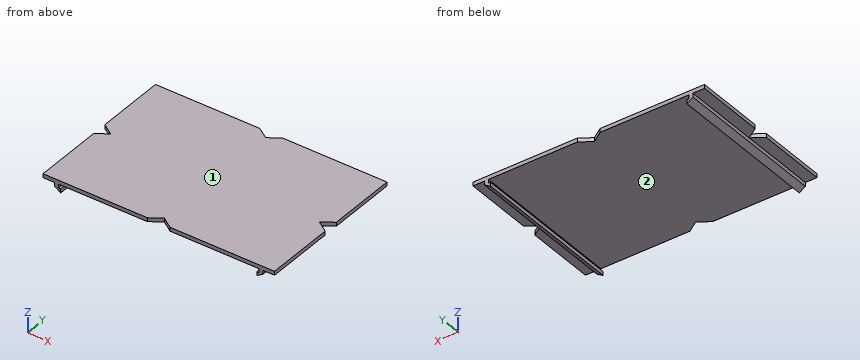
```python
from build123d import *

# Parameters (mm, degrees)
BOSS_EXTRUDE1_DEPTH = 5
BOSS_EXTRUDE2_DEPTH = 200


with BuildPart() as part:
    # Sketch1 → Boss-Extrude1 (new body)
    with BuildSketch(Plane.XY):
        Polygon((-150, 100), (-150, 9.861218113), (-135.20817283, 0), (-150, -9.861218113), (-150, -100), (-14.79182717, -100), (0, -90.138781887), (14.79182717, -100), (150, -100), (150, -9.861218113), (135.20817283, 0), (150, 9.861218113), (150, 100), (14.79182717, 100), (0, 90.138781887), (-14.79182717, 100), align=None)
    extrude(amount=BOSS_EXTRUDE1_DEPTH)

    # Sketch2 → Boss-Extrude2 (add)
    with BuildSketch(Plane(origin=(0, 100, 0), x_dir=(1, 0, 0), z_dir=(0, 1, 0))):
        Polygon((-135, 0), (-130, 0), (-130, 5), (-127, 5), (-127, 10), (-135, 5), align=None)
    boss_extrude2 = extrude(amount=-BOSS_EXTRUDE2_DEPTH)

    # Mirror1: Boss-Extrude2 across plane
    add(boss_extrude2.mirror(Plane(origin=(0, 0, 0), x_dir=(0, 0, 1), z_dir=(1, 0, 0))))


solid = part.part
```
Geometry check sheet. Reference: the model listing, model coordinates, mm. Face numbers are marked on the shaded views. Give positions to 0.01 mm unless a question says otherwise; leave off trailing zeros. Order: outer loops, then holes, each group sorted by start corner. A loop starts at its lowest first (then second) coordinate and runs counter-clockwise, first axis right, second up. Notation, with made-up numbers: (3.25, -21.5) - (35.25, -21.5) arc R25 cw to (35.25, -0.5) - close; hole circle Ø7 at (15.25, 50). An arc over 180 degrees is marked (long way). Write item = value, one per line. Start each with the question number.
1) Draft check along X on the marked faces 1 and 2. Enter one of: released by +X, released by -X, zero draft, split by the parting line, or undercut.
2) Section check C-C (x = -5.5). Enter the section's corners in (y, z).
3) Scan lines: L1, parallel to Z at x = 126, y = 88.5; L2, parallel to X at y = 52, z = -4.75; L3, parallel to X at y = -52, z = -8.25. Record each from-to range of solid material in increasing order.
4) Section check B-B (x = 58). Enter the section's corners in (y, z), then the cut area to 3 significant figures.
5) Section check A-A (y = 18.5). Enter the section's corners in (x, z).
6) Gauge pin test, flat ends, axial feed: pin 1 Ø5.5 at (y, z) = (29, -7.5) entering from -X; pin 2 Ø5.5 at (y, z) = (-0.5, -1.5) entering from +X; pin 3 Ø1.5 at (y, z) = (21.5, -7.5) entering from +X. Record the tip position at first contact, or that the pin passes through.
Geometry check:
q1.face_1 = zero draft
q1.face_2 = undercut
q2.outline = (-93.81, 0) - (93.81, 0) - (93.81, 5) - (-93.81, 5) - close
q3.L1 = 0 to 5
q3.L2 = -135 to -130, 130 to 135
q3.L3 = -129.8 to -127, 127 to 129.8
q4.outline = (-100, 0) - (100, 0) - (100, 5) - (-100, 5) - close
q4.area = 1,000 mm2
q5.outline = (-150, 0) - (-135, 0) - (-135, -5) - (-127, -10) - (-127, -5) - (-130, -5) - (-130, 0) - (130, 0) - (130, -5) - (127, -5) - (127, -10) - (135, -5) - (135, 0) - (150, 0) - (150, 5) - (-150, 5) - close
q6.pin_1 = -135
q6.pin_2 = 139.42
q6.pin_3 = 132.2
